Study the drawing (mm; zero at the part's minimum x, y, z) and answer. Coordinates: 2 decimals unless noted, no trailing zeros. Order: outer loops, then holes, each group sorted by start corner. A loop starts at its lowest first (then second) coordinate and runs counter-clockwise, first axis right, second up.
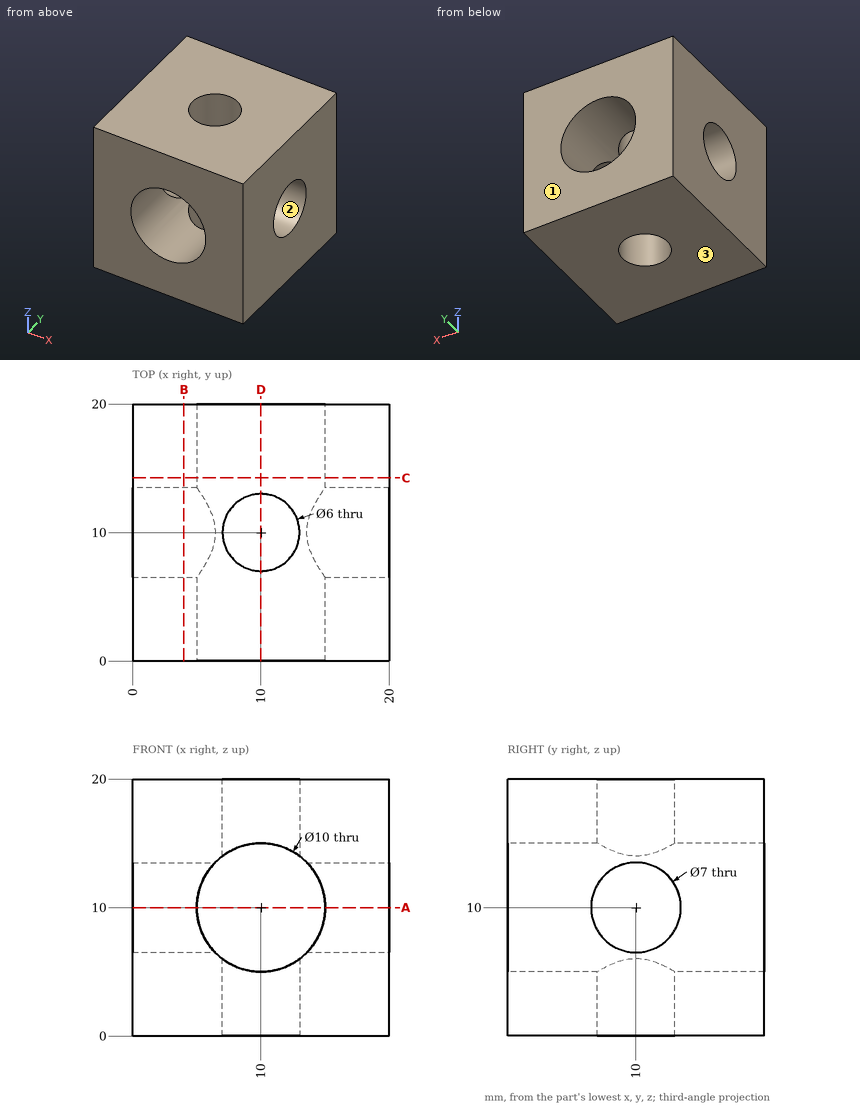
1) A cutting plane is placed at C-C, the plane y = 14.25. Determine the outline of the cut face in (x, z), and give its area (3 significant figures).
A:
outline: (0, 0) - (20, 0) - (20, 20) - (0, 20) - close; hole circle Ø10 at (10, 10)
area: 321 mm2
2) Straight lines are drawn through the part: line 1 (X direction, y = 19, z = 6.5); line 2 (Z direction, x = 9.75, y = 18); line 3 (X direction, y = 2.75, z = 7). For each, find the intervals that lie inside material, in ascending order.
A:
line 1: x = 0 to 6.43, 13.57 to 20
line 2: z = 0 to 5.01, 14.99 to 20
line 3: x = 0 to 6, 14 to 20
3) A cutting plane is placed at A-A, the plane z = 10. Determine the outline of the cut face in (x, y), and give its area (3 significant figures).
A:
outline: (0, 0) - (5, 0) - (5, 6.5) - (0, 6.5) - close; (0, 13.5) - (5, 13.5) - (5, 20) - (0, 20) - close; (15, 0) - (20, 0) - (20, 6.5) - (15, 6.5) - close; (15, 13.5) - (20, 13.5) - (20, 20) - (15, 20) - close
area: 130 mm2
4) Determine the mould class of the marked faces 1, 2 and 3 for opening direction Y: pulls with the +Y half, pulls with the -Y half, needs draft (parallel to the pull), parting line crosses it, or undercut.
A:
face 1: pulls with the +Y half
face 2: undercut
face 3: needs draft
5) A cutting plane is placed at D-D, the plane x = 10. Determine the outline of the cut face in (y, z).
A:
outline: (0, 0) - (7, 0) - (7, 5) - (0, 5) - close; (0, 15) - (7, 15) - (7, 20) - (0, 20) - close; (13, 0) - (20, 0) - (20, 5) - (13, 5) - close; (13, 15) - (20, 15) - (20, 20) - (13, 20) - close
6) A cutting plane is placed at B-B, the plane x = 4. Determine the outline of the cut face in (y, z).
A:
outline: (0, 0) - (20, 0) - (20, 20) - (0, 20) - close; hole circle Ø7 at (10, 10)
7) A flat-ended cylindrical pin translates along its axis: pin 1 Ø4 at (y, z) = (10, 10) entering from +X. Find the tip coordinate at first contact, or state that the pin passes through.
A:
pin 1: passes through
